```python
from build123d import *

# Parameters (mm, degrees)
F0_R     = 27.94
F0_R_2   = 3.37312
F0_R_3   = 9.779
F1_DEPTH = 31.75
F2_R     = 15.5575
F2_R_2   = 12.3825
F3_DEPTH = 1.778


with BuildPart() as f1:
    # F0 (on Front) → F1 (new body)
    with BuildSketch(Plane.XZ):
        Circle(F0_R)
        with Locations((0, -19.90725)):
            Circle(F0_R_2, mode=Mode.SUBTRACT)
        with Locations((-19.90725, 0)):
            Circle(F0_R_2, mode=Mode.SUBTRACT)
        Circle(F0_R_3, mode=Mode.SUBTRACT)
        with Locations((19.90725, 0)):
            Circle(F0_R_2, mode=Mode.SUBTRACT)
        with Locations((0, 19.90725)):
            Circle(F0_R_2, mode=Mode.SUBTRACT)
    extrude(amount=F1_DEPTH)

    # F2 (on Front) → F3 (cut)
    with BuildSketch(Plane.XZ):
        Circle(F2_R)
        Circle(F2_R_2, mode=Mode.SUBTRACT)
    extrude(amount=F3_DEPTH, mode=Mode.SUBTRACT)


solid = f1.part
```
Source: CAD feature listing. Evaluate the final solid. Frame: model axes, mm. A direction names the side the tool comes from. Coordinates: 2 decimals unless noted, no trailing zeros. Write each loop counter-clockwise with the first axis right and the second up, starting at its lowest first coordinate (ties: lowest second). Pieces come first, ordered by that corner, then holes. Notation, with made-up numbers: (47.25, -18.75) - (102.25, -18.75) arc R23 cw to (102.25, -2.75) - close; hole circle Ø6 at (80, -5.75). An arc over 180 degrees is marked (long way). Answer as a JSON object with one key per item and string values.
Q1. Draft query along Z for faces 1 (the cylindrical face through (-3.64, -15.65, 27.7)), 2 (the cylindrical face through (-3.37, -0.88, -15.19)), 3 (the flat face through (12, 0, -12)). Return one class per face: released by +Z, released by -Z, zero draft, split by the parting line, or undercut.
Ans:
{"face 1": "split by the parting line", "face 2": "undercut", "face 3": "zero draft"}
Q2. Section query B-B, the plane x = 0. Output: boundary loops of the cut face in (y, z), plus the area to 3 significant figures.
Ans:
{"outline": "(-31.75, -27.94) - (0, -27.94) - (0, -23.28) - (-31.75, -23.28) - close; (-31.75, -16.53) - (0, -16.53) - (0, -15.56) - (-1.78, -15.56) - (-1.78, -12.38) - (0, -12.38) - (0, -9.78) - (-31.75, -9.78) - close; (-31.75, 9.78) - (0, 9.78) - (0, 12.38) - (-1.78, 12.38) - (-1.78, 15.56) - (0, 15.56) - (0, 16.53) - (-31.75, 16.53) - close; (-31.75, 23.28) - (0, 23.28) - (0, 27.94) - (-31.75, 27.94) - close", "area": "714 mm2"}
Q3. Section query D-D, the plane z = 19. Output: boundary loops of the cut face in (x, y).
Ans:
{"outline": "(-20.49, -31.75) - (-3.25, -31.75) - (-3.25, 0) - (-20.49, 0) - close; (3.25, -31.75) - (20.49, -31.75) - (20.49, 0) - (3.25, 0) - close"}
Q4. Set-up query: faces 4 (the cylindrical face through (11.81, -0.88, 3.72)), 5 (the cylindrical face through (23.125, -15.653, 1.013)). Return all of +Z, -Z, +X, -X, +Y, -Y with unobstructed straight access to the full face (end or side cutting, diameter ignored); none if empty.
Ans:
{"face 4": "+Y", "face 5": "+Y, -Y"}
Q5. First-contact query: pin 1 Ø1 at (x, y) = (-0.5, -23) entering from +Z; pin 2 Ø3 at (x, y) = (11, -14) entering from +Z; pin 3 Ø3 at (x, y) = (-6.5, -18.5) entering from +Z. Flat tips, straight axial feed; report the tip coordinate or a pass-through.
Ans:
{"pin 1": "stops at z = 27.94", "pin 2": "stops at z = 26.28", "pin 3": "stops at z = 27.49"}
Q6. Section query A-A, the plane z = 0. Output: boundary loops of the cut face in (x, y), plus the area to 3 significant figures.
Ans:
{"outline": "(-27.94, -31.75) - (-23.28, -31.75) - (-23.28, 0) - (-27.94, 0) - close; (-16.53, -31.75) - (-9.78, -31.75) - (-9.78, 0) - (-12.38, 0) - (-12.38, -1.78) - (-15.56, -1.78) - (-15.56, 0) - (-16.53, 0) - close; (9.78, -31.75) - (16.53, -31.75) - (16.53, 0) - (15.56, 0) - (15.56, -1.78) - (12.38, -1.78) - (12.38, 0) - (9.78, 0) - close; (23.28, -31.75) - (27.94, -31.75) - (27.94, 0) - (23.28, 0) - close", "area": "714 mm2"}
Q7. Material intervals for line 1 (Z direction, x = 0, y = -12); line 2 (Z direction, x = 0, y = -1.5); line 3 (X direction, y = -25, z = 2.5), sorted ascending. Write a range as [from, to].
Ans:
{"line 1": "z = [-27.94, -23.28], [-16.53, -9.78], [9.78, 16.53], [23.28, 27.94]", "line 2": "z = [-27.94, -23.28], [-16.53, -15.56], [-12.38, -9.78], [9.78, 12.38], [15.56, 16.53], [23.28, 27.94]", "line 3": "x = [-27.83, -22.17], [-17.64, -9.45], [9.45, 17.64], [22.17, 27.83]"}
Q8. Section query C-C, the plane x = 18.5. Output: boundary loops of the cut face in (y, z).
Ans:
{"outline": "(-31.75, -20.94) - (0, -20.94) - (0, -3.07) - (-31.75, -3.07) - close; (-31.75, 3.07) - (0, 3.07) - (0, 20.94) - (-31.75, 20.94) - close"}
